from build123d import *

# Parameters (mm, degrees)
F0_W      = 104.648
F0_H      = 88.9
F1_DEPTH  = 12.7
F2_W      = 69.596
F2_H      = 6.35
F3_DEPTH  = 28.575
F4_W      = 69.596
F4_H      = 6.35
F5_DEPTH  = 28.575
F10_DEPTH = 1.524
F11_W     = 31.242
F11_H     = 31.75
F12_DEPTH = 28.449
F14_W     = 6.35
F14_H     = 11.049
F15_DEPTH = 35.053
F17_W     = 6.35
F17_H     = 11.049
F20_DEPTH = 35.053
F19_W     = 6.35
F19_H     = 11.049
F21_DEPTH = 35.053
F22_W     = 6.35
F22_H     = 11.049
F23_DEPTH = 35.053
F25_DEPTH = 26.925
F27_DEPTH = 20.575
F29_DEPTH = 20.575


with BuildPart() as f1:
    # F0 (on Front) → F1 (new body, symmetric)
    with BuildSketch(Plane.XZ):
        Rectangle(F0_W, F0_H)
    extrude(amount=F1_DEPTH, both=True)

    # F2 (on face) → F3 (cut)
    with BuildSketch(Plane.XY.offset(44.45)):
        with Locations((-17.526, 9.525)):
            Rectangle(F2_W, F2_H)
        Polygon((-45.974, -1.524), (-52.324, -1.524), (-52.324, -12.7), (17.272, -12.7), (17.272, -6.35), (-45.974, -6.35), align=None)
    extrude(amount=-F3_DEPTH, mode=Mode.SUBTRACT)

    # F4 (on face) → F5 (cut)
    with BuildSketch(Plane(origin=(0, 0, -44.45), x_dir=(1, 0, 0), z_dir=(0, 0, -1))):
        Polygon((-45.974, 6.35), (17.272, 6.35), (17.272, 12.7), (-52.324, 12.7), (-52.324, 1.524), (-45.974, 1.524), align=None)
        with Locations((-17.526, -9.525)):
            Rectangle(F4_W, F4_H)
    extrude(amount=-F5_DEPTH, mode=Mode.SUBTRACT)

    # F9 (on face) + F7 (on face) → F10 (join, symmetric)
    with BuildSketch(Plane(origin=(0, 12.7, 0), x_dir=(-1, 0, 0), z_dir=(0, 1, 0))):
        Polygon((52.324, 15.875), (-17.272, 15.875), (-52.324, 15.875), (-52.324, -15.875), (-17.272, -15.875), (52.324, -15.875), align=None)
    with BuildSketch(Plane.XZ.offset(12.7)):
        Polygon((52.324, -15.875), (52.324, 15.875), (17.272, 15.875), (-52.324, 15.875), (-52.324, -15.875), (17.272, -15.875), align=None)
    extrude(amount=F10_DEPTH, both=True, dir=(0, 1, 0))

    # F11 (on face) → F12 (cut, through all)
    with BuildSketch(Plane.XZ.offset(14.224)):
        with Locations((36.703, 0)):
            Rectangle(F11_W, F11_H)
    extrude(amount=-F12_DEPTH, mode=Mode.SUBTRACT)

    # F14 (on face) → F15 (cut, through all)
    with BuildSketch(Plane(origin=(17.272, 0, 0), x_dir=(0, -1, 0), z_dir=(-1, 0, 0))):
        with Locations((9.525, 21.3995)):
            Rectangle(F14_W, F14_H)
    extrude(amount=-F15_DEPTH, mode=Mode.SUBTRACT)

    # F17 (on face) → F20 (cut, through all)
    with BuildSketch(Plane(origin=(17.272, 0, 0), x_dir=(0, -1, 0), z_dir=(-1, 0, 0))):
        with Locations((-9.525, 21.3995)):
            Rectangle(F17_W, F17_H)
    extrude(amount=-F20_DEPTH, mode=Mode.SUBTRACT)

    # F19 (on face) → F21 (cut, through all)
    with BuildSketch(Plane(origin=(17.272, 0, 0), x_dir=(0, -1, 0), z_dir=(-1, 0, 0))):
        with Locations((-9.525, -21.3995)):
            Rectangle(F19_W, F19_H)
    extrude(amount=-F21_DEPTH, mode=Mode.SUBTRACT)

    # F22 (on face) → F23 (cut, through all)
    with BuildSketch(Plane(origin=(17.272, 0, 0), x_dir=(0, -1, 0), z_dir=(-1, 0, 0))):
        with Locations((9.525, -21.3995)):
            Rectangle(F22_W, F22_H)
    extrude(amount=-F23_DEPTH, mode=Mode.SUBTRACT)

    # F24 (on face) → F25 (cut, through all)
    with BuildSketch(Plane.XZ.offset(12.7)):
        Polygon((52.324, 26.924), (52.324, 44.45), (34.798, 26.924), align=None)
        Polygon((34.798, -26.924), (52.324, -44.45), (52.324, -26.924), align=None)
    extrude(amount=-F25_DEPTH, mode=Mode.SUBTRACT)

    # F26 (on face) → F27 (cut, through all)
    with BuildSketch(Plane.XZ.offset(6.35)):
        Polygon((23.749, -15.875), (34.798, -26.924), (52.324, -26.924), (52.324, -15.875), align=None)
        Polygon((52.324, 26.924), (34.798, 26.924), (23.749, 15.875), (52.324, 15.875), align=None)
    extrude(amount=-F27_DEPTH, mode=Mode.SUBTRACT)

    # F28 (on face) → F29 (cut, through all)
    with BuildSketch(Plane.XZ.offset(6.35)):
        with BuildLine():
            ThreePointArc((-26.289, -24.5745), (-22.3376873067, -26.2111873067), (-20.701, -30.1625))
            ThreePointArc((-20.701, -30.1625), (-22.3376873067, -34.1138126933), (-26.289, -35.7505))
            Line((-26.289, -35.7505), (-2.413, -35.7505))
            ThreePointArc((-2.413, -35.7505), (-8.001, -30.1625), (-2.413, -24.5745))
            Line((-2.413, -24.5745), (-26.289, -24.5745))
        make_face()
        with BuildLine():
            ThreePointArc((-26.289, -35.7505), (-22.3376873067, -34.1138126933), (-20.701, -30.1625))
            ThreePointArc((-20.701, -30.1625), (-22.3376873067, -26.2111873067), (-26.289, -24.5745))
            ThreePointArc((-26.289, -24.5745), (-31.877, -30.1625), (-26.289, -35.7505))
        make_face()
        with BuildLine():
            ThreePointArc((3.175, -30.1625), (1.5383126933, -26.2111873067), (-2.413, -24.5745))
            ThreePointArc((-2.413, -24.5745), (-8.001, -30.1625), (-2.413, -35.7505))
            ThreePointArc((-2.413, -35.7505), (1.5383126933, -34.1138126933), (3.175, -30.1625))
        make_face()
        with BuildLine():
            ThreePointArc((-26.289, 35.7505), (-22.3376873067, 34.1138126933), (-20.701, 30.1625))
            ThreePointArc((-20.701, 30.1625), (-22.3376873067, 26.2111873067), (-26.289, 24.5745))
            Line((-26.289, 24.5745), (-2.413, 24.5745))
            ThreePointArc((-2.413, 24.5745), (-8.001, 30.1625), (-2.413, 35.7505))
            Line((-2.413, 35.7505), (-26.289, 35.7505))
        make_face()
        with BuildLine():
            ThreePointArc((-26.289, 24.5745), (-22.3376873067, 26.2111873067), (-20.701, 30.1625))
            ThreePointArc((-20.701, 30.1625), (-22.3376873067, 34.1138126933), (-26.289, 35.7505))
            ThreePointArc((-26.289, 35.7505), (-31.877, 30.1625), (-26.289, 24.5745))
        make_face()
        with BuildLine():
            ThreePointArc((3.175, 30.1625), (1.5383126933, 34.1138126933), (-2.413, 35.7505))
            ThreePointArc((-2.413, 35.7505), (-8.001, 30.1625), (-2.413, 24.5745))
            ThreePointArc((-2.413, 24.5745), (1.5383126933, 26.2111873067), (3.175, 30.1625))
        make_face()
    extrude(amount=-F29_DEPTH, mode=Mode.SUBTRACT)


solid = f1.part
Source: CAD feature listing. Evaluate the final solid. Frame: model axes, mm. A direction names the side the tool comes from. Coordinates: 2 decimals unless noted, no trailing zeros. Order: outer loops, then holes, each group sorted by start corner. A loop starts at its lowest first (then second) coordinate and runs counter-clockwise, first axis right, second up.
Item 1: Cut plane B-B (x = -1). Return loops of the section in (y, z) (3 decimals), plus the area to 3 significant figures.
Output values:
outline: (-14.224, -15.875) - (-6.35, -15.875) - (-6.35, -24.756) - (6.35, -24.756) - (6.35, -15.875) - (14.224, -15.875) - (14.224, 15.875) - (6.35, 15.875) - (6.35, 24.756) - (-6.35, 24.756) - (-6.35, 15.875) - (-14.224, 15.875) - close; (-6.35, -44.45) - (6.35, -44.45) - (6.35, -35.569) - (-6.35, -35.569) - close; (-6.35, 35.569) - (6.35, 35.569) - (6.35, 44.45) - (-6.35, 44.45) - close
area: 1,350 mm2
Item 2: First-contact query: P1, Ø1.9, axis at x = -50.5, z = -32.5, coming from the -Y side; P2, Ø10, axis at x = -8.5, z = 24, coming from the +Y side; P3, Ø2.5, axis at y = -3, z = 33, coming from the -X side. Flat tips, straight axial feed; report the tip coordinate or a pass-through.
Output values:
P1: stops at y = -1.52
P2: stops at y = 6.35
P3: stops at x = -45.97
Item 3: Set-up query: faces 1 (the face through (-31.876, -0.089, 30.285)), 2 (the face through (41.412, -0.178, 33.538)), 3 (the face through (26, 10, -26.924)). Return all of +Z, -Z, +X, -X, +Y, -Y with unobstructed straight access to the full face (end or side cutting, diameter ignored); none if empty.
Output values:
face 1: +Y, -Y
face 2: +X, +Y, -Y
face 3: +X, -X, +Y
Item 4: Cut plane D-D (y = -9.5). Return loops of the section in (x, z) (3 decimals), plus the area to 3 significant figures.
Output values:
outline: (-52.324, -15.875) - (21.082, -15.875) - (21.082, 15.875) - (-52.324, 15.875) - close; (17.272, -44.45) - (52.324, -44.45) - (34.798, -26.924) - (17.272, -26.924) - close; (17.272, 26.924) - (34.798, 26.924) - (52.324, 44.45) - (17.272, 44.45) - close
area: 3,250 mm2
Item 5: Cut plane A-A (y = 1.75). Count the separate pieces of the cut face and the enclosed holes in it, plus the area to 3 significant figures.
Output values:
separate pieces: 1
enclosed holes: 2
area: 6,760 mm2
Item 6: Material intervals for line 1 (Z direction, x = -30, y = -4); line 2 (Z direction, x = 32.5, y = -12.25); line 3 (Z direction, x = -1, y = 6.75) (3 decimals), sorted ascending.
Output values:
line 1: z = -44.45 to -34.34, -25.98 to 25.98, 34.34 to 44.45
line 2: z = -44.45 to -26.92, 26.92 to 44.45
line 3: z = -15.875 to 15.875
Item 7: Pull-direction query (Z, two-part tool) for faces 4 (the face through (31, -12.7, 36)), 5 (the face through (26, -9, 26.924)); classes: pulls with the +Z half, pulls with the -Z half, needs draft (parallel to the pull), parting line crosses it, or undercut.
Output values:
face 4: needs draft
face 5: undercut
Item 8: Cut plane C-C (x = 39). Return loops of the section in (y, z).
Output values:
outline: (-12.7, -44.45) - (12.7, -44.45) - (12.7, -31.13) - (-12.7, -31.13) - close; (-12.7, 31.13) - (12.7, 31.13) - (12.7, 44.45) - (-12.7, 44.45) - close
